Solid Edge part; units mm, degrees
sketch "Sketch1" plane through (0, 0, 0) normal (0, 0, 1) x (1, 0, 0)
  line L0 (0.457, 8.85) -> (0.6095, 8.85)
  line L1 (0.6095, 8.85) -> (0.762, 11.75)
  line L2 (0.762, 11.75) -> (0.762, 13.188)
  line L3 (0.762, 13.188) -> (0.6095, 14.65)
  line L4 (0.6095, 14.65) -> (0.457, 14.65)
  line L5 (0.457, 14.65) -> (0.5333, 13.2)
  line L6 (0.5333, 13.2) -> (0.457, 11.75)
  line L7 (0.457, 11.75) -> (0.457, 8.85)
revolve "RevolvedProtrusion1" add sketch "Sketch1" angle 360 about axis through (0.6095, 0, 0) along (-1, 0, 0)
properties material "Steel"
Design review of the part built by this model. Coordinates are the model's own, in mm. Give positions to 0.01 mm unless a question says otherwise; leave off trailing zeros. Order: outer loops, then holes, each group sorted by start corner. A loop starts at its lowest first (then second) coordinate and runs counter-clockwise, first axis right, second up. Notation, with made-up numbers: (-35.5, -14.5) -> (-16.5, -14.5) arc R35 ccw to (-16.5, 20.5) -> close; hole circle Ø10 at (73, 55.25). An arc over 180 degrees is marked (long way). Write each question's results on one line, items separated by ' | '. Start each with the question number.
Q1. Mouldability with a two-part tool opening along Z and no side actions: class faces 1 (the flat face through (0.762, -9, 8)), 2 (the conical face through (0.62, 4.86, 7.62)) as +Z half, -Z half, draft (parallel to the pull), parting line (faces both ways), or undercut.
Q2. Add section A-A on y = 0. Give the boundary of the cut face in (x, z), and give its area (3 significant figures).
Q3. Wall thickness on L1, parallel to X at y = -13, z = -3.5; L2, parallel to X at y = 11, z = -6: over which ranges is each line inside the solid? List them lowest first. Write a range as from..to.
Found:
1) face 1: draft | face 2: undercut
2) outline: (0.46, -14.65) -> (0.61, -14.65) -> (0.76, -13.19) -> (0.76, -11.75) -> (0.61, -8.85) -> (0.46, -8.85) -> (0.46, -11.75) -> (0.53, -13.2) -> close; (0.46, 8.85) -> (0.61, 8.85) -> (0.76, 11.75) -> (0.76, 13.19) -> (0.61, 14.65) -> (0.46, 14.65) -> (0.53, 13.2) -> (0.46, 11.75) -> close | area: 2.65 mm2
3) L1: x = 0.52..0.73 | L2: x = 0.5..0.76
